Drawing for the job (mm, zero at the part's lowest x, y, z). A direction names the side the tool comes from. Coordinates: 2 decimals unless noted, no trailing zeros. Loops run counter-clockwise (first coordinate to the right, second up) from the corner with the lowest first, then second, coordinate; pieces in that order, holes last. Notation, with made-up numbers: (31.25, 44.5) -> (67.25, 44.5) arc R10 ccw to (67.25, 50.5) -> close; hole circle Ø7 at (65.5, 35.25). An arc over 180 degrees is marked (long way). Write each question's results on one line, items separated by ' | '.
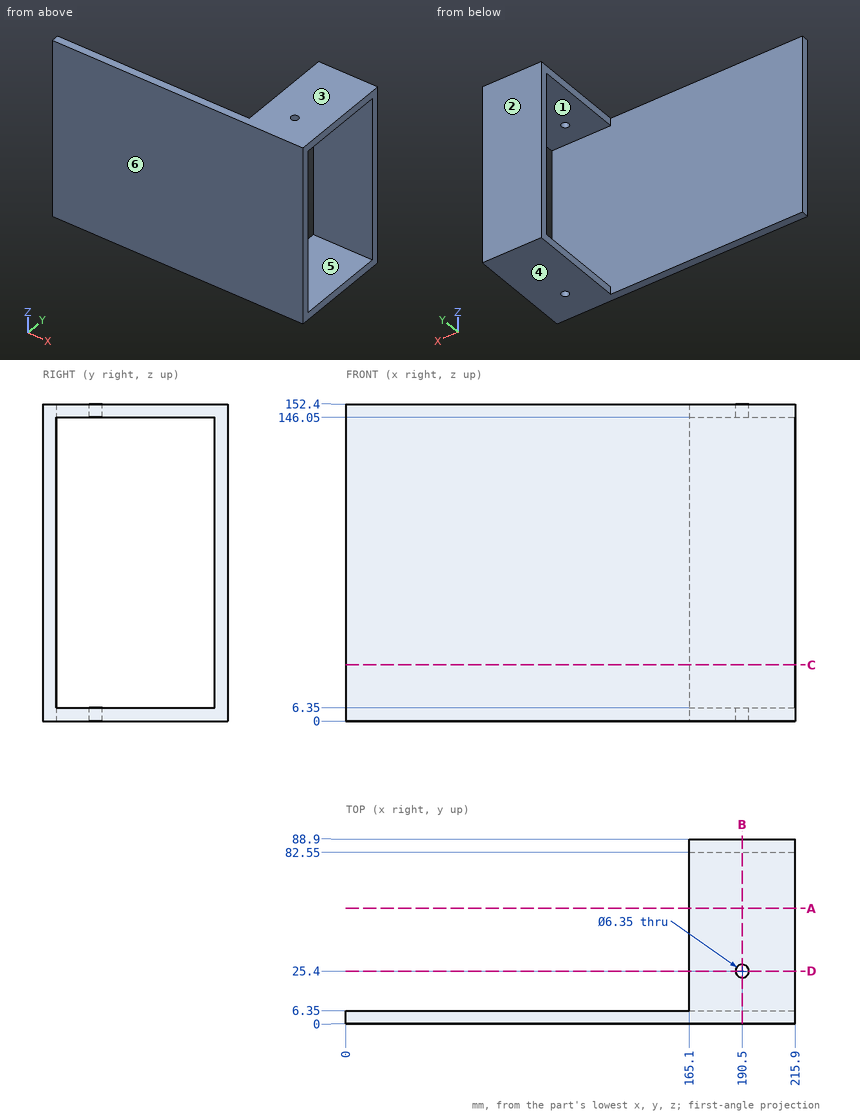
1) Slice it at B-B (x = 190.5). Write the cut outline in (y, z) (3 decimals).
Outcome:
outline: (0, 0) -> (22.225, 0) -> (22.225, 6.35) -> (6.35, 6.35) -> (6.35, 146.05) -> (22.225, 146.05) -> (22.225, 152.4) -> (0, 152.4) -> close; (28.575, 0) -> (88.9, 0) -> (88.9, 152.4) -> (28.575, 152.4) -> (28.575, 146.05) -> (82.55, 146.05) -> (82.55, 6.35) -> (28.575, 6.35) -> close
2) Two-plate mould, pull along Z, no slides. Class the marked faces 3, 4, 5 and 6: pulls with the +Z half, pulls with the -Z half, needs draft (parallel to the pull), parting line crosses it, or undercut.
Outcome:
face 3: pulls with the +Z half | face 4: pulls with the -Z half | face 5: undercut | face 6: needs draft
3) Slice it at C-C (z = 27). Write the cut outline in (x, y), then the cut area to 3 significant figures.
Outcome:
outline: (0, 0) -> (215.9, 0) -> (215.9, 6.35) -> (0, 6.35) -> close; (165.1, 82.55) -> (215.9, 82.55) -> (215.9, 88.9) -> (165.1, 88.9) -> close | area: 1,690 mm^2
4) Slice it at A-A (y = 55.5). Write the cut outline in (x, z).
Outcome:
outline: (165.1, 0) -> (215.9, 0) -> (215.9, 6.35) -> (165.1, 6.35) -> close; (165.1, 146.05) -> (215.9, 146.05) -> (215.9, 152.4) -> (165.1, 152.4) -> close
5) Which spindle directions (+Z, -Z, +X, -X, +Y, -Y) get a long thin tool onto all of the face, cutting with end or side? Do the marked faces 1 and 2. Say none if no direction does.
Outcome:
face 1: +X, -X | face 2: +Z, -Z, +X, -X, +Y
6) Drill centre lines: L1, parallel to X at y = 25, z = 3; L2, parallel to Y at x = 190.5, z = 4.5 (3 decimals); L3, parallel to Y at x = 190, z = 149. Where is each one in solid material? Low to high. Write a range as from..to.
Outcome:
L1: x = 165.1..187.35, 193.65..215.9 | L2: y = 0..22.225, 28.575..88.9 | L3: y = 0..22.26, 28.54..88.9
7) Slice it at D-D (y = 25.4). Write the cut outline in (x, z) (3 decimals), then the cut area to 3 significant figures.
Outcome:
outline: (165.1, 0) -> (187.325, 0) -> (187.325, 6.35) -> (165.1, 6.35) -> close; (165.1, 146.05) -> (187.325, 146.05) -> (187.325, 152.4) -> (165.1, 152.4) -> close; (193.675, 0) -> (215.9, 0) -> (215.9, 6.35) -> (193.675, 6.35) -> close; (193.675, 146.05) -> (215.9, 146.05) -> (215.9, 152.4) -> (193.675, 152.4) -> close | area: 565 mm^2
8) Pin check, flat tips, straight feed: pin 1 (8 mm diameter, centred on x = 140, z = 112, fed in from -Y); pin 2 (5 mm diameter, centred on x = 113, z = 47, fed in from +Y); pin 3 (4 mm diameter, centred on x = 190.5, y = 25.4, fed in from -Z). Stop position of each tip, or through.
Outcome:
pin 1: stops at y = 0 | pin 2: stops at y = 6.35 | pin 3: passes through
